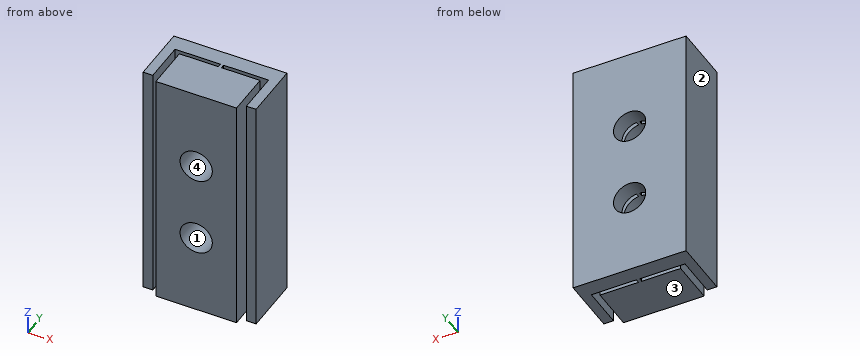
from build123d import *

# Parameters (mm, degrees)
SKETCH_1_W          = 5
SKETCH_1_H          = 15
EXTRUDE_1_DEPTH     = 3
EXTRUDE_2_DEPTH     = 15
SKETCH_3_R          = 1
CUT_EXTRUDE_1_DEPTH = 5
SKETCH_5_W          = 2.409632894
SKETCH_5_H          = 0.246400488
SKETCH_5_W_2        = 2.393250689
CUT_EXTRUDE_3_DEPTH = 15
SKETCH_6_W          = 0.6
SKETCH_6_H          = 0.4
CUT_EXTRUDE_4_DEPTH = 15


with BuildPart() as part:
    # 草图1 → 凸台-拉伸1 (new body)
    with BuildSketch(Plane(origin=(0, 0, 0), x_dir=(1, 0, 0), z_dir=(0, 1, 0))):
        with Locations((-2.5, -7.5)):
            Rectangle(SKETCH_1_W, SKETCH_1_H)
    extrude(amount=EXTRUDE_1_DEPTH)

    # 草图2 → 凸台-拉伸2 (add)
    with BuildSketch(Plane(origin=(0, 0, 0), x_dir=(-1, 0, 0), z_dir=(0, 0, -1))):
        Polygon((-0.4, 0), (-0.4, 3), (5.4, 3), (5.4, 0), (6, 0), (6, 4), (-1, 4), (-1, 0), align=None)
    extrude(amount=-EXTRUDE_2_DEPTH)

    # 草图3 → 切除-拉伸1 (cut, through all)
    with BuildSketch(Plane(origin=(0, 4, 0), x_dir=(1, 0, 0), z_dir=(0, 1, 0))):
        with Locations((-2.5, -10)):
            Circle(SKETCH_3_R)
        with Locations((-2.5, -5)):
            Circle(SKETCH_3_R)
    extrude(amount=-CUT_EXTRUDE_1_DEPTH, mode=Mode.SUBTRACT)

    # 草图5 → 切除-拉伸3 (cut)
    with BuildSketch(Plane.XY.offset(15)):
        with Locations((-3.795183553, 2.876799756)):
            Rectangle(SKETCH_5_W, SKETCH_5_H)
        with Locations((-1.196625345, 2.876799756)):
            Rectangle(SKETCH_5_W_2, SKETCH_5_H)
    extrude(amount=-CUT_EXTRUDE_3_DEPTH, mode=Mode.SUBTRACT)

    # 草图6 → 切除-拉伸4 (cut)
    with BuildSketch(Plane(origin=(0, 0, 0), x_dir=(-1, 0, 0), z_dir=(0, 0, -1))):
        with Locations((-0.7, 0.2)):
            Rectangle(SKETCH_6_W, SKETCH_6_H)
        with Locations((5.7, 0.2)):
            Rectangle(SKETCH_6_W, SKETCH_6_H)
    extrude(amount=-CUT_EXTRUDE_4_DEPTH, mode=Mode.SUBTRACT)


solid = part.part
Source: CAD feature listing. Evaluate the final solid. Frame: model axes, mm. Face numbers are marked on the shaded views. Give positions to 0.01 mm unless a question says otherwise; leave off trailing zeros. Write each loop counter-clockwise with the first axis right and the second up, starting at its lowest first coordinate (ties: lowest second). Pieces come first, ordered by that corner, then holes. Notation, with made-up numbers: (26, -16.75) -> (39, -16.75) arc R5 ccw to (39, -7.75) -> close; hole circle Ø3 at (82.5, 18). An arc over 180 degrees is marked (long way). Return JSON: item names as keys, results as strings. Group by question number.
1. Section D-D, the plane z = 1. Output: boundary loops of the cut face in (x, y), then the cut area to 3 significant figures.
2. Mould query, pull axis X, two halves, no side actions, for the marked faces 1, 2, 3 and 4. Classes: +X half, -X half, draft (parallel to the pull), parting line (faces both ways), or undercut.
3. Section A-A, the plane z = 5. Output: boundary loops of the cut face in (x, y).
4. Section B-B, the plane x = -4. Output: boundary loops of the cut face in (y, z), then the cut area to 3 significant figures.
5. Section C-C, the plane y = 2.2. Output: boundary loops of the cut face in (x, z).
6. Material intervals for line 1 (Z direction, x = -2.5, y = 2.7); line 2 (X direction, y = 1.9, z = 2.75); line 3 (X direction, y = 0.8, z = 5), sorted ascending. Write a range as from..to.
Determined:
{
 "1": {"outline": "(-6, 0.4) -> (-5.4, 0.4) -> (-5.4, 3) -> (-2.59, 3) -> (-2.59, 2.75) -> (-5, 2.75) -> (-5, 0) -> (0, 0) -> (0, 2.75) -> (-2.39, 2.75) -> (-2.39, 3) -> (0.4, 3) -> (0.4, 0.4) -> (1, 0.4) -> (1, 4) -> (-6, 4) -> close", "area": "23.9 mm2"},
 "2": {"face 1": "undercut", "face 2": "-X half", "face 3": "draft", "face 4": "undercut"},
 "3": {"outline": "(-6, 0.4) -> (-5.4, 0.4) -> (-5.4, 3) -> (-3.5, 3) -> (-3.5, 4) -> (-6, 4) -> close; (-5, 0) -> (-3.5, 0) -> (-3.5, 2.75) -> (-5, 2.75) -> close; (-1.5, 0) -> (0, 0) -> (0, 2.75) -> (-1.5, 2.75) -> close; (-1.5, 3) -> (0.4, 3) -> (0.4, 0.4) -> (1, 0.4) -> (1, 4) -> (-1.5, 4) -> close"},
 "4": {"outline": "(0, 0) -> (2.75, 0) -> (2.75, 15) -> (0, 15) -> close; (3, 0) -> (4, 0) -> (4, 15) -> (3, 15) -> close", "area": "56.3 mm2"},
 "5": {"outline": "(-6, 0) -> (-5.4, 0) -> (-5.4, 15) -> (-6, 15) -> close; (-5, 0) -> (0, 0) -> (0, 15) -> (-5, 15) -> close; (0.4, 0) -> (1, 0) -> (1, 15) -> (0.4, 15) -> close; hole circle Ø2 at (-2.5, 5); hole circle Ø2 at (-2.5, 10)"},
 "6": {"line 1": "z = 0..4, 6..9, 11..15", "line 2": "x = -6..-5.4, -5..0, 0.4..1", "line 3": "x = -6..-5.4, -5..-3.5, -1.5..0, 0.4..1"}
}
